Could you check a few things on this model? Use its own coordinates, in mm. A direction names the side the tool comes from. Round coordinates to 2 decimals unless told otherwise and drop trailing zeros. Write each loop counter-clockwise with the first axis right and the second up, starting at its lowest first coordinate (ties: lowest second). Pieces come first, ordered by that corner, then holes. Notation, with made-up numbers: (-27.5, 14) -> (16.5, 14) arc R34 cw to (16.5, 47) -> close; hole circle Ø11 at (72.5, 16). An arc over 180 degrees is marked (long way). Answer as CSV lines item,"result". Start each with the question number.
Q1. Imagine slicing it at A-A on x = 19. Please give me the cut outline in (y, z), and give its area (3 significant figures).
Q2. For faces 5 (the flat face through (7.65, 21, 13)), 6 (the flat face through (18, 4.309, -1)), 7 (the flat face through (9.65, 0, -1)), 8 (the flat face through (8, 29.309, -35)), 9 (the flat face through (9.65, 38, -1)), which set-ups out of +Z, -Z, +X, -X, +Y, -Y let a thin tool reach every point of the face, with its end or its side?
Q3. Imagine slicing it at B-B on x = -0.5. Please give me the cut outline in (y, z), and give its area (3 significant figures).
Q4. If I drill on line 1 (Y direction, x = 6.9, z = -14); line 2 (Z direction, x = 26.5, y = 13); line 3 (Y direction, x = 0.5, z = -24), over which ranges is the centre line in solid material (lowest first)? Write a range as [from, to].
Q5. If we mould it in two halves opening along Y, with no side actions, what happens to faces 1 (the flat face through (2, -5.221, -1)), 2 (the flat face through (8, 6.309, -65)), 3 (the flat face through (4, 39, -80)), 4 (the flat face through (0, 41.839, -1))? For each: pulls with the +Y half, pulls with the -Y half, needs draft (parallel to the pull), parting line crosses it, or undercut.
Q6. Will these pins go through, and if not, where does the flat tip stop? pin 1 Ø1 at (x, y) = (7, 22.5) entering from +Z; pin 2 Ø3 at (y, z) = (2, -35) entering from +X; pin 3 Ø6 at (y, z) = (33, 57) entering from -X.
from build123d import *

# Parameters (mm, degrees)
BOSS_EXTRU_1_DEPTH      = 80
BOSS_EXTRU_1_DEPTH_BACK = 80
ESQUISSE4_R             = 1.5
ESQUISSE4_W             = 23
ESQUISSE4_H             = 12.2
ENL_V_MAT_EXTRU_1_DEPTH = 95
ENL_V_START             = -2
ESQUISSE5_W             = 5
ESQUISSE5_H             = 12.2
ESQUISSE5_R             = 1.5
ENL_V_MAT_EXTRU_2_DEPTH = 2
BOSS_EXTRU_3_DEPTH      = 50
BOSS_EXTRU_3_DEPTH_BACK = 50
CHANFREIN2_SIZE         = 2
ESQUISSE11_W            = 30
ESQUISSE11_H            = 20
ENL_V_MAT_EXTRU_4_DEPTH = 11
ENL_V_MAT_EXTRU_5_DEPTH = 8


with BuildPart() as part:
    # Esquisse1 → Boss.-Extru.1 (new, two sides: drawn at the far end of the back side and taken through both)
    with BuildSketch(Plane.XY.offset(-BOSS_EXTRU_1_DEPTH_BACK)):
        Polygon((-2.561538462, -0.921153846), (-2.561538462, 1.078846154), (-5.65, 1.078846154), (-5.65, -5.221153846), (5.65, -5.221153846), (9.45, -5.221153846), (9.65, -5.221153846), (9.65, 43.838846154), (9.45, 43.838846154), (5.65, 43.838846154), (-5.65, 43.838846154), (-5.65, 37.538846154), (-2.561538462, 37.538846154), (-2.561538462, 39.538846154), (-3.15, 39.538846154), (-3.15, 41.838846154), (3.15, 41.838846154), (3.15, 39.538846154), (2.061538462, 39.538846154), (2.061538462, 37.538846154), (5.65, 37.538846154), (5.65, 1.078846154), (2.061538462, 1.078846154), (2.061538462, -0.921153846), (3.15, -0.921153846), (3.15, -3.221153846), (-3.15, -3.221153846), (-3.15, -0.921153846), align=None)
    extrude(amount=BOSS_EXTRU_1_DEPTH + BOSS_EXTRU_1_DEPTH_BACK)

    # Esquisse4 → Enlèv. mat.-Extru.1 (cut)
    with BuildSketch(Plane.ZY.offset(-5.65)):
        with Locations((-14, 19.308846154)):
            Circle(ESQUISSE4_R)
        with Locations(Location((14, 19.308846154, 0), (0, 0, 270))):
            Circle(ESQUISSE4_R)
        with Locations((0, 19.308846154)):
            Rectangle(ESQUISSE4_W, ESQUISSE4_H)
    extrude(amount=-ENL_V_MAT_EXTRU_1_DEPTH, mode=Mode.SUBTRACT)

    # Esquisse5 → Enlèv. mat.-Extru.2 (cut)
    # profile 1 of 2: a face of its own
    with BuildSketch(Plane(origin=(9.65, 0, 0), x_dir=(0, 0, -1), z_dir=(1, 0, 0)).offset(ENL_V_START)):
        with Locations((14, 19.308846154)):
            Rectangle(ESQUISSE5_W, ESQUISSE5_H)
        with Locations(Location((14, 19.308846154, 0), (0, 0, 180))):
            Circle(ESQUISSE5_R, mode=Mode.SUBTRACT)
    # profile 2 of 2: a face of its own
    with BuildSketch(Plane(origin=(9.65, 0, 0), x_dir=(0, 0, -1), z_dir=(1, 0, 0)).offset(ENL_V_START)):
        with Locations((-14, 19.308846154)):
            Rectangle(ESQUISSE5_W, ESQUISSE5_H)
        with Locations(Location((-14, 19.308846154, 0), (0, 0, 90))):
            Circle(ESQUISSE5_R, mode=Mode.SUBTRACT)
    extrude(amount=ENL_V_MAT_EXTRU_2_DEPTH, mode=Mode.SUBTRACT)

    # Esquisse9 → Boss.-Extru.3 (add, two sides: drawn at the far end of the back side and taken through both)
    with BuildSketch(Plane.XY.offset(-BOSS_EXTRU_3_DEPTH_BACK)):
        Polygon((23.35, 4.308846154), (27.35, 4.308846154), (27.35, 8.308846154), (27.35, 30.308846154), (27.35, 34.308846154), (9.65, 34.308846154), (9.65, 30.308846154), (23.35, 30.308846154), (23.35, 8.308846154), (9.65, 8.308846154), (9.65, 4.308846154), align=None)
    extrude(amount=BOSS_EXTRU_3_DEPTH + BOSS_EXTRU_3_DEPTH_BACK)

    # Chanfrein2
    # the kernel refuses this chamfer: 2 mm, written as the material it adds along each edge
    with BuildSketch(Plane(origin=(23.35, 8.308846154, 50), x_dir=(-0.9996219169112968, -0.027495876610587375, 0), z_dir=(0, 0, -1)), Plane(origin=(9.65, 4.308846154, -50), x_dir=(-0.027495876610585623, -0.9996219169112968, 0), z_dir=(0, 0, 1))) as chanfrein2_piece_1:
        Polygon((CHANFREIN2_SIZE * 0.999621916911, CHANFREIN2_SIZE * 0.0274958766106), (-CHANFREIN2_SIZE * 0.0274958766106, CHANFREIN2_SIZE * 0.999621916911), (0, 0), align=None)
    extrude(amount=100)
    with BuildSketch(Plane(origin=(23.35, 30.308846154, 50), x_dir=(-0.9996219169112968, 0.027495876610585647, 0), z_dir=(0, 0, -1)), Plane(origin=(9.65, 30.308846154, 50), x_dir=(-0.027495876610588235, -0.9996219169112968, 0), z_dir=(0, 0, -1)), Plane(origin=(9.65, 34.308846154, -50), x_dir=(-0.02749587661058651, 0.9996219169112968, 0), z_dir=(0, 0, 1)), Plane(origin=(9.65, 8.308846154, -50), x_dir=(-0.02749587661058651, 0.9996219169112968, 0), z_dir=(0, 0, 1))) as chanfrein2_piece_2:
        Polygon((CHANFREIN2_SIZE * 0.999621916911, -CHANFREIN2_SIZE * 0.0274958766106), (-CHANFREIN2_SIZE * 0.0274958766106, -CHANFREIN2_SIZE * 0.999621916911), (0, 0), align=None)
    extrude(amount=100)
    with BuildSketch(Plane(origin=(5.65, 37.538846154, -80), x_dir=(-0.9996219169112968, 0.02749587661058563, 0), z_dir=(0, 0, 1)), Plane(origin=(5.65, 1.078846154, -80), x_dir=(0.027495876610586504, 0.9996219169112968, 0), z_dir=(0, 0, 1))) as chanfrein2_piece_3:
        Polygon((CHANFREIN2_SIZE * 0.999621916911, CHANFREIN2_SIZE * 0.0274958766106), (-CHANFREIN2_SIZE * 0.0274958766106, CHANFREIN2_SIZE * 0.999621916911), (0, 0), align=None)
    extrude(amount=160)
    # the kernel refuses this chamfer: 2 mm, written as the material it takes off along each edge
    with BuildSketch(Plane(origin=(-2.561538462, 1.078846154, -85.143365976), x_dir=(-0.9996219169112968, 0.027495876610586716, 0), z_dir=(0, 0, 1)), Plane(origin=(-5.65, 1.078846154, -85.143365976), x_dir=(-0.027495876610586487, -0.9996219169112968, 0), z_dir=(0, 0, 1)), Plane(origin=(-5.65, -5.221153846, -85.143365976), x_dir=(0.9996219169112968, -0.027495876610586494, 0), z_dir=(0, 0, 1)), Plane(origin=(9.65, -5.221153846, -85.143365976), x_dir=(0.027495876610586494, 0.9996219169112968, 0), z_dir=(0, 0, 1)), Plane(origin=(9.65, 43.838846154, -85.143365976), x_dir=(-0.9996219169112968, 0.027495876610585623, 0), z_dir=(0, 0, 1)), Plane(origin=(-5.65, 37.538846154, -85.143365976), x_dir=(0.999621916911297, -0.027495876610582174, 0), z_dir=(0, 0, 1)), Plane(origin=(-5.65, 43.838846154, -85.143365976), x_dir=(-0.02749587661058651, -0.9996219169112968, 0), z_dir=(0, 0, 1))) as chanfrein2_2_piece_1:
        Polygon((CHANFREIN2_SIZE * 0.999621916911, CHANFREIN2_SIZE * 0.0274958766106), (-CHANFREIN2_SIZE * 0.0274958766106, CHANFREIN2_SIZE * 0.999621916911), (0, 0), align=None)
    extrude(amount=170.286731952, mode=Mode.SUBTRACT)
    with BuildSketch(Plane(origin=(27.35, 4.308846154, -55.143365976), x_dir=(0.027495876610585623, 0.9996219169112968, 0), z_dir=(0, 0, 1)), Plane(origin=(27.35, 34.308846154, -55.143365976), x_dir=(-0.9996219169112968, 0.027495876610585647, 0), z_dir=(0, 0, 1))) as chanfrein2_2_piece_2:
        Polygon((CHANFREIN2_SIZE * 0.999621916911, CHANFREIN2_SIZE * 0.0274958766106), (-CHANFREIN2_SIZE * 0.0274958766106, CHANFREIN2_SIZE * 0.999621916911), (0, 0), align=None)
    extrude(amount=110.286731952, mode=Mode.SUBTRACT)

    # Esquisse11 → Enlèv. mat.-Extru.4 (cut)
    with BuildSketch(Plane.ZY.offset(-5.65)):
        Polygon((-50, 29.308846154), (-50, 32.308846154), (-80, 32.308846154), (-80, 6.308846154), (-50, 6.308846154), (-50, 9.308846154), align=None)
        Polygon((80, 32.308846154), (50, 32.308846154), (50, 29.308846154), (50, 9.308846154), (50, 6.308846154), (80, 6.308846154), align=None)
        with Locations((-35, 19.308846154)):
            Rectangle(ESQUISSE11_W, ESQUISSE11_H)
        with Locations((35, 19.308846154)):
            Rectangle(ESQUISSE11_W, ESQUISSE11_H)
    extrude(amount=-ENL_V_MAT_EXTRU_4_DEPTH, mode=Mode.SUBTRACT)

    # Esquisse12 → Enlèv. mat.-Extru.5 (cut)
    with BuildSketch(Plane(origin=(27.35, 0, 0), x_dir=(0, 0, -1), z_dir=(1, 0, 0))):
        Polygon((20, 28.308846154), (10, 28.308846154), (-10, 28.308846154), (-20.122761397, 28.308846154), (-20.122761397, 10.308846154), (-10, 10.308846154), (10, 10.308846154), (20, 10.308846154), align=None)
    extrude(amount=-ENL_V_MAT_EXTRU_5_DEPTH, mode=Mode.SUBTRACT)


solid = part.part
Checks:
1,outline,"(4.31, -50) -> (8.31, -50) -> (8.31, 50) -> (4.31, 50) -> close; (30.31, -50) -> (34.31, -50) -> (34.31, 50) -> (30.31, 50) -> close"
1,area,"800 mm^2"
2,face 5,"+X"
2,face 6,"+Z, -Z, +X, -Y"
2,face 7,"+X, -Y"
2,face 8,"-Z, -X"
2,face 9,"+X, +Y"
3,outline,"(-5.22, -80) -> (-3.22, -80) -> (-3.22, 80) -> (-5.22, 80) -> close; (41.84, -80) -> (43.84, -80) -> (43.84, 80) -> (41.84, 80) -> close"
3,area,"640 mm^2"
4,line 1,"[-5.22, 17.81], [20.81, 43.84]"
4,line 2,"[-50, -20], [20.12, 50]"
4,line 3,"[-5.22, -3.22], [41.84, 43.84]"
5,face 1,"pulls with the -Y half"
5,face 2,"undercut"
5,face 3,"needs draft"
5,face 4,"undercut"
6,pin 1,"z = 20"
6,pin 2,"x = 10.84"
6,pin 3,"x = 5.19"
